Autodesk Inventor part; units mm, degrees
ref_plane "YZ Plane" through (0, 0, 0) normal (1, 0, 0) x (0, 1, 0)
ref_plane "XZ Plane" through (0, 0, 0) normal (0, 1, 0) x (-1, 0, 0)
ref_plane "XY Plane" through (0, 0, 0) normal (0, 0, 1) x (1, 0, 0)
sketch "Sketch1" plane through (0, 0, 0) normal (0, 0, 1) x (1, 0, 0)
  line L0 (104.168, 1.684) -> (710.4569, 587.1704)
  arc A0 (100, 0) -> (104.168, 1.684) centre (100, 6) ccw
  line L1 (0, 0) -> (100, 0)
  dimension "d25" = 6
  dimension "d48" = 710.457
  dimension "d49" = 136
  dimension "d50" = 100
contour flange "Contour Flange1" sketch "Sketch1" thickness 3 bend radius 3 width 980 along (0, 0, 1) mid plane no both sides no wall seen from (50, 0, 0) lies toward (0, 1, 0) curves L1 A0 L0
bend "Bend1"
corner "Corner1"
mirror "Mirror1" about plane through (0, 0, 0) normal (1, 0, 0)
equation "\"d25\" = Thickness + BendRadius"
equation "\"d7\" = Thickness"
equation "\"d8\" = BendReliefWidth"
equation "\"d9\" = BendReliefDepth"
equation "\"d10\" = MinimumRemnant"
equation "\"d11\" = TransitionRadius"
equation "\"d13\" = BendRadius"
equation "\"d15\" = CornerReliefSize"
equation "\"d16\" = GapSize"
equation "\"d17\" = JacobiRadiusSize"
equation "\"BendRadius\" = Thickness"
equation "\"BendReliefWidth\" = Thickness"
equation "\"BendReliefDepth\" = 0.5 * Thickness"
equation "\"CornerReliefSize\" = 4 * Thickness"
equation "\"MinimumRemnant\" = 2 * Thickness"
equation "\"TransitionRadius\" = BendRadius"
equation "\"JacobiRadiusSize\" = BendRadius"
equation "\"GapSize\" = Thickness"
equation "\"d38\" = d40 + d44"
equation "\"d39\" = d40"
equation "\"d44\" = d40"
properties part number "MSC 041 sheet belly main" material "Stainless Steel"
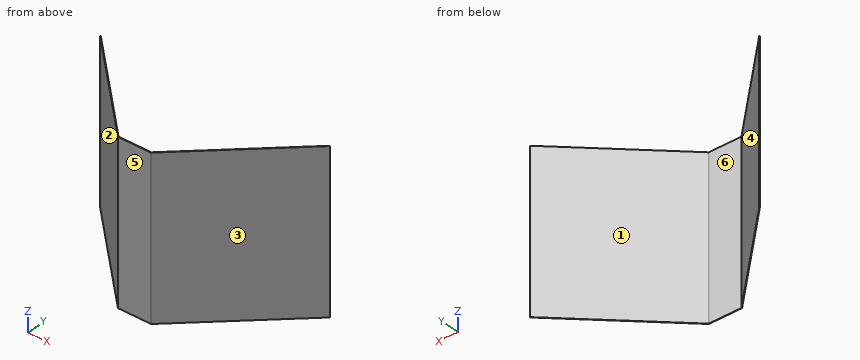
Could you check a few things on this model? Use its own coordinates, in mm. Face numbers are marked on the shaded views. A direction names the side the tool comes from. Coordinates: 2 decimals unless noted, no trailing zeros. Order: outer loops, then holes, each group sorted by start corner. A loop starts at its lowest first (then second) coordinate and runs counter-clockwise, first axis right, second up. Notation, with made-up numbers: (79.25, -12.5) -> (118.25, -12.5) arc R26 cw to (118.25, 9.5) -> close; hole circle Ø10 at (58.25, -36). An arc over 180 degrees is marked (long way). One line per item, written item: value. Start each with the question number.
1) Which directions (+Z, -Z, +X, -X, +Y, -Y) give clear straight access to the entire face, cutting with the end or side of a thin tool? Please do the marked faces 1 and 2.
2) Imagine slicing it at C-C on x = 44. List the corners of the cut face in (y, z) for me, plus the area to 3 significant figures.
3) I'm going to push flat-ended pins straight in: pin 1 (5 mm diameter, centred on x = -186.5, z = 211.5, fed in from +Y); pin 2 (1 mm diameter, centred on x = -499.5, z = 200, fed in from +Y) (3 decimals); pin 3 (1 mm diameter, centred on x = -442.5, z = 559, fed in from +Y). Where does each tip first touch, or does it pass through?
4) Imagine slicing it at B-B on y = 128. List the corners of the cut face in (x, z) for me, plus the area to 3 significant figures.
5) Imagine slicing it at A-A on z = 810. List the corners of the cut face in (x, y) for me.
6) We'd pull the mould along X, two halves only. Please class the marked faces 3, 4, 5 and 6: +X half, -X half, draft (parallel to the pull), parting line (faces both ways), or undercut.
7) If I drill on L1, parallel to X at y = 342, z = 445.5; L2, parallel to X at y = 390, z = 125.5; L3, parallel to Y at x = 17, z = 59.5, over which ranges is the centre line in solid material (lowest first)? Write a range as [from, to].
8) Imagine slicing it at D-D on x = 581. List the corners of the cut face in (y, z) for me.
Answer list:
1. face 1: +Z, -Z, +Y
1. face 2: +Z, -Z, -X, -Y
2. outline: (0, 0) -> (3, 0) -> (3, 980) -> (0, 980) -> close
2. area: 2,940 mm2
3. pin 1: stops at y = 87.78
3. pin 2: stops at y = 388.105
3. pin 3: stops at y = 333.06
4. outline: (-234.97, 0) -> (-230.65, 0) -> (-230.65, 980) -> (-234.97, 980) -> close; (230.65, 0) -> (234.97, 0) -> (234.97, 980) -> (230.65, 980) -> close
4. area: 8,460 mm2
5. outline: (-710.46, 587.17) -> (-104.17, 1.68) arc R6 ccw to (-100, 0) -> (100, 0) arc R6 ccw to (104.17, 1.68) -> (710.46, 587.17) -> (708.37, 589.33) -> (102.08, 3.84) arc R3 cw to (100, 3) -> (-100, 3) arc R3 cw to (-102.08, 3.84) -> (-708.37, 589.33) -> close
6. face 3: +X half
6. face 4: undercut
6. face 5: draft
6. face 6: undercut
7. L1: x = [-456.58, -452.26], [452.26, 456.58]
7. L2: x = [-506.28, -501.96], [501.96, 506.28]
7. L3: y = [0, 3]
8. outline: (462.16, 0) -> (466.33, 0) -> (466.33, 980) -> (462.16, 980) -> close
